CAD build for the part. Positions are in the model's coordinates, mm. A direction names the side the tool comes from. Coordinates: 2 decimals unless noted, no trailing zeros. Order: outer loops, then holes, each group sorted by start corner. A loop starts at its lowest first (then second) coordinate and runs counter-clockwise, first axis right, second up. Notation, with made-up numbers: (44, 58) - (98, 58) arc R20 ccw to (98, 69) - close; hole circle Ø3 at (62.5, 50). An arc over 180 degrees is marked (long way). Return JSON: item names as keys, results as strings.
from build123d import *

# Parameters (mm, degrees)
CYLINDER016_R          = 2
CYLINDER016_DEPTH      = 2
CYLINDER012_R          = 2
CYLINDER012_DEPTH      = 2
CYLINDER015_R          = 2
CYLINDER015_DEPTH      = 2
CYLINDER017_R          = 2
CYLINDER017_DEPTH      = 2
CYLINDER013_R          = 2
CYLINDER013_DEPTH      = 2
CYLINDER014_R          = 2
CYLINDER014_DEPTH      = 2
CYLINDER018_R          = 2
CYLINDER018_DEPTH      = 2
CYLINDER019_R          = 2
CYLINDER019_DEPTH      = 2
CYLINDER020_R          = 2
CYLINDER020_DEPTH      = 2
CYLINDER011_R          = 2
CYLINDER011_DEPTH      = 2
BOX003_W               = 18.5
BOX003_H               = 50
BOX003_DEPTH           = 10
CYLINDER010_R          = 1
CYLINDER010_DEPTH      = 5
CYLINDER008_R          = 1.15
CYLINDER008_DEPTH      = 5
CYLINDER006_R          = 1.15
CYLINDER006_DEPTH      = 5
CYLINDER009_R          = 1.15
CYLINDER009_DEPTH      = 5
CYLINDER007_R          = 1.15
CYLINDER007_DEPTH      = 5
CYLINDER001_R          = 1.15
CYLINDER001_DEPTH      = 5
CYLINDER002_R          = 1.15
CYLINDER002_DEPTH      = 5
CYLINDER003_R          = 1.15
CYLINDER003_DEPTH      = 5
CYLINDER004_R          = 1.15
CYLINDER004_DEPTH      = 5
CYLINDER005_R          = 1.15
CYLINDER005_DEPTH      = 5
CYLINDER_R             = 1.15
CYLINDER_DEPTH         = 5
BOX001_W               = 334.204
BOX001_H               = 140.47
BOX001_DEPTH           = 1.5
FILLET001_R            = 5
BOX_W                  = 330.204
BOX_H                  = 136.47
BOX_DEPTH              = 10.5
FILLET_R               = 5
BOX002_W               = 344.204
BOX002_H               = 150.47
BOX002_DEPTH           = 15.5
FILLET002_R            = 1
FILLET003_R            = 1
CUT005_PLACEMENT_ANGLE = 180


with BuildPart() as cylinder016:
    # Cylinder016 → Cylinder016 (new body)
    with BuildSketch(Plane(origin=(23.5, 27.36, 0), x_dir=(1, 0, 0), z_dir=(0, 0, 1))):
        Circle(CYLINDER016_R)
    extrude(amount=CYLINDER016_DEPTH)


with BuildPart() as cylinder012:
    # Cylinder012 → Cylinder012 (new body)
    with BuildSketch(Plane(origin=(-153.35, 56.36, 0), x_dir=(1, 0, 0), z_dir=(0, 0, 1))):
        Circle(CYLINDER012_R)
    extrude(amount=CYLINDER012_DEPTH)


with BuildPart() as cylinder015:
    # Cylinder015 → Cylinder015 (new body)
    with BuildSketch(Plane(origin=(-23.5, 27.36, 0), x_dir=(1, 0, 0), z_dir=(0, 0, 1))):
        Circle(CYLINDER015_R)
    extrude(amount=CYLINDER015_DEPTH)


with BuildPart() as cylinder017:
    # Cylinder017 → Cylinder017 (new body)
    with BuildSketch(Plane(origin=(153.352, -56.36, 0), x_dir=(1, 0, 0), z_dir=(0, 0, 1))):
        Circle(CYLINDER017_R)
    extrude(amount=CYLINDER017_DEPTH)


with BuildPart() as cylinder013:
    # Cylinder013 → Cylinder013 (new body)
    with BuildSketch(Plane(origin=(-20, -23.36, 0), x_dir=(1, 0, 0), z_dir=(0, 0, 1))):
        Circle(CYLINDER013_R)
    extrude(amount=CYLINDER013_DEPTH)


with BuildPart() as cylinder014:
    # Cylinder014 → Cylinder014 (new body)
    with BuildSketch(Plane(origin=(-20, -56.36, 0), x_dir=(1, 0, 0), z_dir=(0, 0, 1))):
        Circle(CYLINDER014_R)
    extrude(amount=CYLINDER014_DEPTH)


with BuildPart() as cylinder018:
    # Cylinder018 → Cylinder018 (new body)
    with BuildSketch(Plane(origin=(153.352, 56.36, 0), x_dir=(1, 0, 0), z_dir=(0, 0, 1))):
        Circle(CYLINDER018_R)
    extrude(amount=CYLINDER018_DEPTH)


with BuildPart() as cylinder019:
    # Cylinder019 → Cylinder019 (new body)
    with BuildSketch(Plane(origin=(20, -23.36, 0), x_dir=(1, 0, 0), z_dir=(0, 0, 1))):
        Circle(CYLINDER019_R)
    extrude(amount=CYLINDER019_DEPTH)


with BuildPart() as cylinder020:
    # Cylinder020 → Cylinder020 (new body)
    with BuildSketch(Plane(origin=(20, -56.36, 0), x_dir=(1, 0, 0), z_dir=(0, 0, 1))):
        Circle(CYLINDER020_R)
    extrude(amount=CYLINDER020_DEPTH)


with BuildPart() as fusion001:
    # Cylinder011 → Cylinder011 (new body)
    with BuildSketch(Plane(origin=(-153.35, -56.36, 0), x_dir=(1, 0, 0), z_dir=(0, 0, 1))):
        Circle(CYLINDER011_R)
    extrude(amount=CYLINDER011_DEPTH)

    # Fusion001: union Cylinder016, Cylinder012, Cylinder015, Cylinder017, Cylinder013, Cylinder014, Cylinder018, Cylinder019, Cylinder020
    add(cylinder016.part)
    add(cylinder012.part)
    add(cylinder015.part)
    add(cylinder017.part)
    add(cylinder013.part)
    add(cylinder014.part)
    add(cylinder018.part)
    add(cylinder019.part)
    add(cylinder020.part)


with BuildPart() as cube003:
    # Box003 → Box003 (new body)
    with BuildSketch(Plane(origin=(-9.25, -75.25, 2), x_dir=(1, 0, 0), z_dir=(0, 0, 1))):
        with Locations((9.25, 25)):
            Rectangle(BOX003_W, BOX003_H)
    extrude(amount=BOX003_DEPTH)


with BuildPart() as cylinder010:
    # Cylinder010 → Cylinder010 (new body)
    with BuildSketch(Plane(origin=(0, -19.14, 0), x_dir=(1, 0, 0), z_dir=(0, 0, 1))):
        Circle(CYLINDER010_R)
    extrude(amount=CYLINDER010_DEPTH)


with BuildPart() as cylinder008:
    # Cylinder008 → Cylinder008 (new body)
    with BuildSketch(Plane(origin=(-23.5, 27.36, 0), x_dir=(1, 0, 0), z_dir=(0, 0, 1))):
        Circle(CYLINDER008_R)
    extrude(amount=CYLINDER008_DEPTH)


with BuildPart() as cylinder006:
    # Cylinder006 → Cylinder006 (new body)
    with BuildSketch(Plane(origin=(-20, -23.36, 0), x_dir=(1, 0, 0), z_dir=(0, 0, 1))):
        Circle(CYLINDER006_R)
    extrude(amount=CYLINDER006_DEPTH)


with BuildPart() as cylinder009:
    # Cylinder009 → Cylinder009 (new body)
    with BuildSketch(Plane(origin=(23.5, 27.36, 0), x_dir=(1, 0, 0), z_dir=(0, 0, 1))):
        Circle(CYLINDER009_R)
    extrude(amount=CYLINDER009_DEPTH)


with BuildPart() as cylinder007:
    # Cylinder007 → Cylinder007 (new body)
    with BuildSketch(Plane(origin=(20, -23.36, 0), x_dir=(1, 0, 0), z_dir=(0, 0, 1))):
        Circle(CYLINDER007_R)
    extrude(amount=CYLINDER007_DEPTH)


with BuildPart() as cylinder001:
    # Cylinder001 → Cylinder001 (new body)
    with BuildSketch(Plane(origin=(153.35, -56.36, 0), x_dir=(1, 0, 0), z_dir=(0, 0, 1))):
        Circle(CYLINDER001_R)
    extrude(amount=CYLINDER001_DEPTH)


with BuildPart() as cylinder002:
    # Cylinder002 → Cylinder002 (new body)
    with BuildSketch(Plane(origin=(-153.35, 56.36, 0), x_dir=(1, 0, 0), z_dir=(0, 0, 1))):
        Circle(CYLINDER002_R)
    extrude(amount=CYLINDER002_DEPTH)


with BuildPart() as cylinder003:
    # Cylinder003 → Cylinder003 (new body)
    with BuildSketch(Plane(origin=(-153.35, -56.36, 0), x_dir=(1, 0, 0), z_dir=(0, 0, 1))):
        Circle(CYLINDER003_R)
    extrude(amount=CYLINDER003_DEPTH)


with BuildPart() as cylinder004:
    # Cylinder004 → Cylinder004 (new body)
    with BuildSketch(Plane(origin=(-20, -56.36, 0), x_dir=(1, 0, 0), z_dir=(0, 0, 1))):
        Circle(CYLINDER004_R)
    extrude(amount=CYLINDER004_DEPTH)


with BuildPart() as cylinder005:
    # Cylinder005 → Cylinder005 (new body)
    with BuildSketch(Plane(origin=(20, -56.36, 0), x_dir=(1, 0, 0), z_dir=(0, 0, 1))):
        Circle(CYLINDER005_R)
    extrude(amount=CYLINDER005_DEPTH)


with BuildPart() as fusion:
    # Cylinder → Cylinder (new body)
    with BuildSketch(Plane(origin=(153.35, 56.36, 0), x_dir=(1, 0, 0), z_dir=(0, 0, 1))):
        Circle(CYLINDER_R)
    extrude(amount=CYLINDER_DEPTH)

    # Fusion: union Cylinder008, Cylinder006, Cylinder009, Cylinder007, Cylinder001, Cylinder002, Cylinder003, Cylinder004, Cylinder005
    add(cylinder008.part)
    add(cylinder006.part)
    add(cylinder009.part)
    add(cylinder007.part)
    add(cylinder001.part)
    add(cylinder002.part)
    add(cylinder003.part)
    add(cylinder004.part)
    add(cylinder005.part)


with BuildPart() as fillet001:
    # Box001 → Box001 (new body)
    with BuildSketch(Plane(origin=(-167.1, -70.23, 14), x_dir=(1, 0, 0), z_dir=(0, 0, 1))):
        with Locations((167.102, 70.235)):
            Rectangle(BOX001_W, BOX001_H)
    extrude(amount=BOX001_DEPTH)

    # Fillet001
    fillet001_edges = [fillet001.edges().sort_by_distance(p)[0] for p in [
        (-167.1, -70.23, 14.75),
        (-167.1, 70.24, 14.75),
        (167.104, -70.23, 14.75),
        (167.104, 70.24, 14.75),
    ]]
    fillet(fillet001_edges, radius=FILLET001_R)


with BuildPart() as fillet_body:
    # Box → Box (new body)
    with BuildSketch(Plane(origin=(-165.102, -68.23, 5), x_dir=(1, 0, 0), z_dir=(0, 0, 1))):
        with Locations((165.102, 68.235)):
            Rectangle(BOX_W, BOX_H)
    extrude(amount=BOX_DEPTH)

    # Fillet
    fillet_edges = [fillet_body.edges().sort_by_distance(p)[0] for p in [
        (-165.102, -68.23, 10.25),
        (-165.102, 68.24, 10.25),
        (165.102, -68.23, 10.25),
        (165.102, 68.24, 10.25),
    ]]
    fillet(fillet_edges, radius=FILLET_R)


with BuildPart() as cut005:
    # Box002 → Box002 (new body)
    with BuildSketch(Plane(origin=(-172.102, -75.235, 0), x_dir=(1, 0, 0), z_dir=(0, 0, 1))):
        with Locations((172.102, 75.235)):
            Rectangle(BOX002_W, BOX002_H)
    extrude(amount=BOX002_DEPTH)

    # Cut: cut Fillet body
    add(fillet_body.part, mode=Mode.SUBTRACT)

    # Cut001: cut Fillet001
    add(fillet001.part, mode=Mode.SUBTRACT)

    # Cut002: cut Fusion
    add(fusion.part, mode=Mode.SUBTRACT)

    # Cut003: cut Cylinder010
    add(cylinder010.part, mode=Mode.SUBTRACT)

    # Cut004: cut Cube003
    add(cube003.part, mode=Mode.SUBTRACT)

    # Fillet002
    fillet002_edges = [cut005.edges().sort_by_distance(p)[0] for p in [
        (-172.102, -75.235, 7.75),
        (-172.102, 0, 15.5),
        (-172.102, 75.235, 7.75),
        (-172.102, 0, 0),
        (0, -75.235, 0),
        (172.102, -75.235, 7.75),
        (0, -75.235, 15.5),
        (0, 75.235, 15.5),
        (172.102, 0, 15.5),
        (0, 75.235, 0),
        (172.102, 75.235, 7.75),
        (172.102, 0, 0),
    ]]
    fillet(fillet002_edges, radius=FILLET002_R)

    # Fillet003
    fillet003_edges = [cut005.edges().sort_by_distance(p)[0] for p in [
        (-9.25, -71.7325, 12),
        (9.25, -71.7325, 12),
        (9.25, -50.2425, 2),
        (-9.25, -50.2425, 2),
    ]]
    fillet(fillet003_edges, radius=FILLET003_R)

    # Cut005: cut Fusion001
    add(fusion001.part, mode=Mode.SUBTRACT)


with BuildPart() as cut005_1:
    # Cut005 placement: moved
    add(cut005.part.rotate(Axis((0, 0, 0), (0, 0, 1)), CUT005_PLACEMENT_ANGLE))


solid = cut005_1.part
Item 1: Wall check: L1, parallel to Y at x = 20, z = 4.45 (3 decimals); L2, parallel to Y at x = -149, z = 5.25 (3 decimals); L3, parallel to X at y = -8.5, z = 5.5. Give the ranges that are in metal, low to high. Write a range as [from, to].
Findings below:
{"L1": "y = [-75.235, 22.21], [24.51, 55.21], [57.51, 75.235]", "L2": "y = [-75.235, -68.24], [68.23, 75.235]", "L3": "x = [-172.1, -165.1], [165.1, 172.1]"}
Item 2: Drop flat-ended pins along their axis: P1, Ø1.4, axis at x = 20, y = 23.36, coming from the -Z side; P2, Ø8, axis at x = 48, y = -35.5, coming from the +Z side; P3, Ø1.2, axis at x = 154, y = -57, coming from the -Z side; P4, Ø1.5, axis at x = 4, z = 3.5, coming from the +Y side. Give the stop position or say it passes through.
Findings below:
{"P1": "passes through", "P2": "stops at z = 5", "P3": "stops at z = 2", "P4": "stops at y = 25.25"}
Item 3: Band-saw the part on C-C, the plane y = 34.5. List the corners of the cut face in (x, z).
Findings below:
{"outline": "(-172.1, 1) arc R1 ccw to (-171.1, 0) - (171.1, 0) arc R1 ccw to (172.1, 1) - (172.1, 14.5) arc R1 ccw to (171.1, 15.5) - (167.1, 15.5) - (167.1, 14) - (165.1, 14) - (165.1, 5) - (9.25, 5) - (9.25, 3) arc R1 cw to (8.25, 2) - (-8.25, 2) arc R1 cw to (-9.25, 3) - (-9.25, 5) - (-165.1, 5) - (-165.1, 14) - (-167.1, 14) - (-167.1, 15.5) - (-171.1, 15.5) arc R1 ccw to (-172.1, 14.5) - close"}
Item 4: Which spindle directions (+Z, -Z, +X, -X, +Y, -Y) get a long thin tool onto all of the face, cutting with end or side? Do faces 4 (the flat face through (0, 72, 12)), 5 (the flat face through (1, -72, 15.5)), 6 (the flat face through (2, -1, 5)). Say none if no direction does.
Findings below:
{"face 4": "+Y", "face 5": "+Z, +X, -X, +Y, -Y", "face 6": "+Z"}
Item 5: Band-saw the part on D-D, the plane y = 8.5. List the corners of the cut face in (x, z), then the cut area to 3 significant figures.
Findings below:
{"outline": "(-172.1, 1) arc R1 ccw to (-171.1, 0) - (171.1, 0) arc R1 ccw to (172.1, 1) - (172.1, 14.5) arc R1 ccw to (171.1, 15.5) - (167.1, 15.5) - (167.1, 14) - (165.1, 14) - (165.1, 5) - (-165.1, 5) - (-165.1, 14) - (-167.1, 14) - (-167.1, 15.5) - (-171.1, 15.5) arc R1 ccw to (-172.1, 14.5) - close", "area": "1,860 mm²"}
Item 6: Band-saw the part on B-B, the plane z = 7.5. List the corners of the cut face in (x, y) (3 decimals).
Findings below:
{"outline": "(-172.102, -74.235) arc R1 ccw to (-171.102, -75.235) - (171.102, -75.235) arc R1 ccw to (172.102, -74.235) - (172.102, 74.235) arc R1 ccw to (171.102, 75.235) - (9.25, 75.235) - (9.25, 68.23) - (160.102, 68.23) arc R5 cw to (165.102, 63.23) - (165.102, -63.24) arc R5 cw to (160.102, -68.24) - (-160.102, -68.24) arc R5 cw to (-165.102, -63.24) - (-165.102, 63.23) arc R5 cw to (-160.102, 68.23) - (-9.25, 68.23) - (-9.25, 75.235) - (-171.102, 75.235) arc R1 ccw to (-172.102, 74.235) - close"}
Item 7: Mould opens along Y. For faces 1 (the flat face through (172.102, 1, 8)), 2 (the flat face through (2, -68.24, 9)), 3 (the flat face through (2, -75.235, 8)) say: released by +Y, released by -Y, zero draft, split by the parting line, or undercut.
Findings below:
{"face 1": "zero draft", "face 2": "undercut", "face 3": "released by -Y"}
Item 8: Band-saw the part on A-A, the plane x = 131. List the corners of the cut face in (y, z) (3 decimals).
Findings below:
{"outline": "(-75.235, 1) arc R1 ccw to (-74.235, 0) - (74.235, 0) arc R1 ccw to (75.235, 1) - (75.235, 14.5) arc R1 ccw to (74.235, 15.5) - (70.23, 15.5) - (70.23, 14) - (68.23, 14) - (68.23, 5) - (-68.24, 5) - (-68.24, 14) - (-70.24, 14) - (-70.24, 15.5) - (-74.235, 15.5) arc R1 ccw to (-75.235, 14.5) - close"}
